from build123d import *

# Parameters (mm, degrees)
SKETCH1_W           = 10.16
SKETCH1_H           = 86.36
SKETCH1_W_2         = 91.44
SKETCH1_H_2         = 10.16
BOSS_EXTRUDE1_DEPTH = 10.16


with BuildPart() as part:
    # Sketch1 → Boss-Extrude1 (new body)
    with BuildSketch(Plane(origin=(0, 0, 0), x_dir=(1, 0, 0), z_dir=(0, 1, 0))):
        Polygon((-228.6, 205.74), (-137.16, 205.74), (-45.72, 205.74), (45.72, 205.74), (137.16, 205.74), (228.6, 205.74), (320.04, 205.74), (320.04, 129.54), (320.04, 43.18), (320.04, -43.18), (320.04, -129.54), (320.04, -205.74), (228.6, -205.74), (137.16, -205.74), (45.72, -205.74), (-45.72, -205.74), (-137.16, -205.74), (-228.6, -205.74), (-320.04, -205.74), (-320.04, -129.54), (-320.04, -43.18), (-320.04, 43.18), (-320.04, 129.54), (-320.04, 205.74), align=None)
        with Locations((-325.12, 86.36)):
            Rectangle(SKETCH1_W, SKETCH1_H)
        with Locations((-325.12, -86.36)):
            Rectangle(SKETCH1_W, SKETCH1_H)
        with Locations((-182.88, -210.82)):
            Rectangle(SKETCH1_W_2, SKETCH1_H_2)
        with Locations((0, -210.82)):
            Rectangle(SKETCH1_W_2, SKETCH1_H_2)
        with Locations((182.88, -210.82)):
            Rectangle(SKETCH1_W_2, SKETCH1_H_2)
        with Locations((325.12, -86.36)):
            Rectangle(SKETCH1_W, SKETCH1_H)
        with Locations((325.12, 86.36)):
            Rectangle(SKETCH1_W, SKETCH1_H)
        with Locations((-182.88, 210.82)):
            Rectangle(SKETCH1_W_2, SKETCH1_H_2)
        with Locations((0, 210.82)):
            Rectangle(SKETCH1_W_2, SKETCH1_H_2)
        with Locations((182.88, 210.82)):
            Rectangle(SKETCH1_W_2, SKETCH1_H_2)
    extrude(amount=BOSS_EXTRUDE1_DEPTH)


solid = part.part
Work out the finished part from the listing and answer in its coordinate system (mm). Round coordinates to 2 decimals unless told otherwise and drop trailing zeros. Order: outer loops, then holes, each group sorted by start corner. A loop starts at its lowest first (then second) coordinate and runs counter-clockwise, first axis right, second up. Notation, with made-up numbers: M 65.5,-35 L 74.5,-35 A21 cw 74.5,-31 Z; hole C 59,42 d1. An arc over 180 degrees is marked long. Put each result on its own line as item: value. Start each with the question number.
Q1. Straight lines are drawn through the part: L1, parallel to X at y = 4.5, z = -6.5; L2, parallel to Z at x = 233, y = 5. For each, find the intervals that lie inside material, in ascending order. Write a range as [from, to].
Q2. Section A-A, the plane z = -3 is taken. Write down the section's boundary in (x, y), and give its area (3 significant figures).
Q3. Section B-B, the plane x = -260 is taken. Write down the section's boundary in (y, z), and give its area (3 significant figures).
Q4. Flat-ended cylindrical pins translate along their axes: pin 1 (3 mm diameter, centred on y = 5, z = 20, fed in from -X); pin 2 (5 mm diameter, centred on y = 5, z = 210, fed in from -X); pin 3 (3 mm diameter, centred on y = 4, z = -165.5, fed in from +X). Find the tip coordinate at first contact, or state that the pin passes through.
Findings below:
1. L1: x = [-320.04, 320.04]
1. L2: z = [-205.74, 205.74]
2. outline: M -320.04,0 L 320.04,0 L 320.04,10.16 L -320.04,10.16 Z
2. area: 6,500 mm^2
3. outline: M 0,-205.74 L 10.16,-205.74 L 10.16,205.74 L 0,205.74 Z
3. area: 4,180 mm^2
4. pin 1: stops at x = -320.04
4. pin 2: stops at x = -228.6
4. pin 3: stops at x = 320.04
